from build123d import *

# Parameters (mm, degrees)
SKETCH1_W                      = 110
SKETCH1_H                      = 24.85
BOSS_EXTRUDE1_DEPTH            = 6
CHAMFER1_SIZE                  = 6
CBORE_FOR_M4_SHCS1_D           = 4.3
CBORE_FOR_M4_SHCS1_DEPTH       = 10.1
CBORE_FOR_M4_SHCS1_CBORE_D     = 8
CBORE_FOR_M4_SHCS1_CBORE_DEPTH = 4
CBORE_FOR_M4_SHCS1_TIP         = 1.291850331


with BuildPart() as part:
    # Sketch1 → Boss-Extrude1 (new body)
    with BuildSketch(Plane.XY):
        Rectangle(SKETCH1_W, SKETCH1_H)
    extrude(amount=BOSS_EXTRUDE1_DEPTH)

    # Chamfer1
    chamfer1_edges = [part.edges().sort_by_distance(p)[0] for p in [
        (0, -12.425, 0),
        (0, 12.425, 0),
    ]]
    chamfer(chamfer1_edges, length=CHAMFER1_SIZE - 0.0001)  # a hair under: the kernel refuses the full size

    # CBORE for M4 SHCS1
    with Locations(Plane(origin=(0, 0, 0), x_dir=(-1, 0, 0), z_dir=(0, 0, -1))):
        with Locations((-47.5, 0), (-32.5, 0), (50, 0)):
            CounterBoreHole(CBORE_FOR_M4_SHCS1_D / 2, CBORE_FOR_M4_SHCS1_CBORE_D / 2, CBORE_FOR_M4_SHCS1_CBORE_DEPTH, depth=CBORE_FOR_M4_SHCS1_DEPTH)
            with Locations((0, 0, -(CBORE_FOR_M4_SHCS1_DEPTH + CBORE_FOR_M4_SHCS1_TIP / 2))):  # 118° drill point
                Cone(0, CBORE_FOR_M4_SHCS1_D / 2, CBORE_FOR_M4_SHCS1_TIP, mode=Mode.SUBTRACT)


solid = part.part
Work out the finished part from the listing and answer in its coordinate system (mm). A direction names the side the tool comes from. Give positions to 0.01 mm unless a question says otherwise; leave off trailing zeros. Loops run counter-clockwise (first coordinate to the right, second up) from the corner with the lowest first, then second, coordinate; pieces in that order, holes last. Notation, with made-up numbers: (71.25, 70.5) -> (90.25, 70.5) arc R21 cw to (90.25, 82.5) -> close; hole circle Ø3 at (-20, 46). An arc over 180 degrees is marked (long way). Use a Markdown table: item, result. Add a question column.
1) The part is cut by section A-A, the plane y = 0. Determine the outline of the cut face in (x, z).
2) The part is cut by section C-C, the plane z = 2.5. Determine the outline of the cut face in (x, y).
3) Consider line 1 along Y through (x, z) = (-50, 2.85); line 2 along Y through (x, z) = (30.5, 1); line 3 along Y through (x, z) = (-12.5, 1.5). Determine where each line is inside the solid, lowest interval first.
4) The part is cut by section D-D, the plane y = 11. Determine the outline of the cut face in (x, z).
5) Each of these flat-tipped pins is pushed along its axis until it touches: P1, Ø2.5, axis at x = 47, y = 0, coming from the -Z side; P2, Ø5, axis at x = 32.5, y = 0, coming from the -Z side. Where does it stop, or does it pass through?
6) For a pull along Y with two mould halves and no side action, classify faces 1 (the flat face through (-0.77, 9.383, 2.958)), 2 (the cylindrical face through (-47.95, 0.65, 5.01)), 3 (the flat face through (31, -2, 4)), 4 (the flat face through (55, 0, 4)) as +Y half, -Y half, draft (parallel to the pull), parting line (faces both ways), or undercut.
7) Which of the six approach directions +Z, -Z, +X, -X, +Y, -Y give full straight-line access (tool end or side, diameter ignored) to faces 5 (the flat face through (-0.77, -9.383, 2.958)), 6 (the cylindrical face through (51.496, 0.176, 1.972))?
Reported:
| question | item | result |
|---|---|---|
| 1 | outline | (-55, 0) -> (-54, 0) -> (-54, 4) -> (-52.15, 4) -> (-52.15, 6) -> (-55, 6) -> close; (-47.85, 4) -> (-46, 4) -> (-46, 0) -> (28.5, 0) -> (28.5, 4) -> (30.35, 4) -> (30.35, 6) -> (-47.85, 6) -> close; (34.65, 4) -> (36.5, 4) -> (36.5, 0) -> (43.5, 0) -> (43.5, 4) -> (45.35, 4) -> (45.35, 6) -> (34.65, 6) -> close; (49.65, 4) -> (51.5, 4) -> (51.5, 0) -> (55, 0) -> (55, 6) -> (49.65, 6) -> close |
| 2 | outline | (-55, -8.93) -> (55, -8.93) -> (55, 8.93) -> (-55, 8.93) -> close; hole circle Ø8 at (-50, 0); hole circle Ø8 at (32.5, 0); hole circle Ø8 at (47.5, 0) |
| 3 | line 1 | y = -9.28 to -4, 4 to 9.28 |
| 3 | line 2 | y = -7.43 to -3.46, 3.46 to 7.43 |
| 3 | line 3 | y = -7.93 to 7.93 |
| 4 | outline | (-55, 4.57) -> (55, 4.57) -> (55, 6) -> (-55, 6) -> close |
| 5 | P1 | passes through |
| 5 | P2 | stops at z = 4 |
| 6 | face 1 | +Y half |
| 6 | face 2 | undercut |
| 6 | face 3 | undercut |
| 6 | face 4 | draft |
| 7 | face 5 | -Z, +X, -X, -Y |
| 7 | face 6 | -Z |
